Input: part model. Units: mm. Frame: model coordinates. Coordinates: 2 decimals unless noted, no trailing zeros. Loops run counter-clockwise (first coordinate to the right, second up) from the corner with the lowest first, then second, coordinate; pieces in that order, holes last.
```python
from build123d import *

# Parameters (mm, degrees)
BOSS_EXTRUDE1_DEPTH = 300
SKETCH3_R           = 2.25
CUT_EXTRUDE1_DEPTH  = 300
SKETCH6_R           = 2.25
CUT_EXTRUDE2_DEPTH  = 10
SKETCH8_R           = 2.25
CUT_EXTRUDE3_DEPTH  = 10


with BuildPart() as part:
    # Sketch1 → Boss-Extrude1 (new body)
    with BuildSketch(Plane(origin=(0, 0, 0), x_dir=(1, 0, 0), z_dir=(0, 1, 0))):
        Polygon((0, 0), (12.7, 0), (12.7, 2), (2, 2), (2, 12.7), (0, 12.7), align=None)
    extrude(amount=BOSS_EXTRUDE1_DEPTH)

    # Sketch3 → Cut-Extrude1 (cut)
    with BuildSketch(Plane(origin=(0, 0, -2), x_dir=(-1, 0, 0), z_dir=(0, 0, -1))):
        with Locations((-7.35, 275)):
            Circle(SKETCH3_R)
        with Locations((-7.35, 175)):
            Circle(SKETCH3_R)
        with Locations((-7.35, 75)):
            Circle(SKETCH3_R)
    extrude(amount=-CUT_EXTRUDE1_DEPTH, mode=Mode.SUBTRACT)

    # Sketch6 → Cut-Extrude2 (cut)
    with BuildSketch(Plane(origin=(2, 0, 0), x_dir=(0, 0, -1), z_dir=(1, 0, 0))):
        with Locations((7.35, 225)):
            Circle(SKETCH6_R)
        with Locations((7.35, 125)):
            Circle(SKETCH6_R)
        with Locations((7.35, 25)):
            Circle(SKETCH6_R)
    extrude(amount=-CUT_EXTRUDE2_DEPTH, mode=Mode.SUBTRACT)

    # Sketch8 → Cut-Extrude3 (cut)
    with BuildSketch(Plane.XY):
        with Locations((7.94, 253.6)):
            Circle(SKETCH8_R)
        with Locations((7.35, 25)):
            Circle(SKETCH8_R)
    extrude(amount=-CUT_EXTRUDE3_DEPTH, mode=Mode.SUBTRACT)


solid = part.part
```
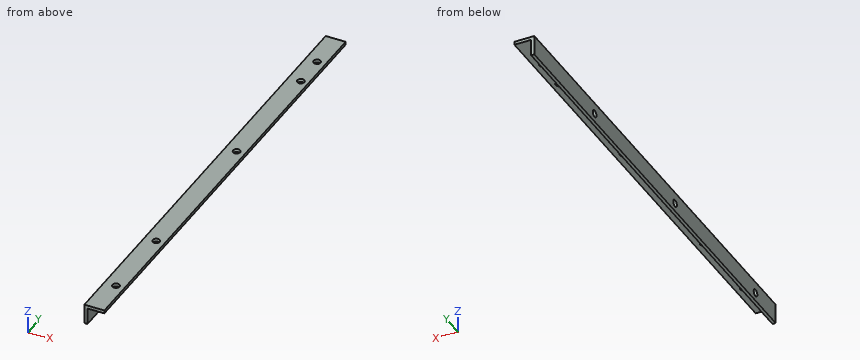
Item 1: Section query A-A (z = -7.35). Output: boundary loops of the cut face in (x, y).
Result:
outline: (0, 0) - (2, 0) - (2, 22.75) - (0, 22.75) - close; (0, 27.25) - (2, 27.25) - (2, 122.75) - (0, 122.75) - close; (0, 127.25) - (2, 127.25) - (2, 222.75) - (0, 222.75) - close; (0, 227.25) - (2, 227.25) - (2, 300) - (0, 300) - close
Item 2: Section query B-B (y = 51). Output: boundary loops of the cut face in (x, z).
Result:
outline: (0, -12.7) - (2, -12.7) - (2, -2) - (12.7, -2) - (12.7, 0) - (0, 0) - close
Item 3: Contact query for flat-ended pins moving along their axis: P1, Ø3, axis at x = 4, z = -10.5, coming from the -Y side; P2, Ø5, axis at x = 7.35, y = 25, coming from the -Z side; P3, Ø5, axis at y = 69, z = -7.5, coming from the +X side. Output: stop coordinate, or through.
Result:
P1: passes through
P2: stops at z = -2
P3: stops at x = 2
Item 4: Line query: L1, parallel to Y at x = 0.5, z = -7.35; L2, parallel to Y at x = 7.35, z = -0.6; L3, parallel to Y at x = 8.75, z = -0.5. Output: solid intervals per line, ascending.
Result:
L1: y = 0 to 22.75, 27.25 to 122.75, 127.25 to 222.75, 227.25 to 300
L2: y = 0 to 22.75, 27.25 to 72.75, 77.25 to 172.75, 177.25 to 251.43, 255.77 to 272.75, 277.25 to 300
L3: y = 0 to 23.24, 26.76 to 73.24, 76.76 to 173.24, 176.76 to 251.5, 255.7 to 273.24, 276.76 to 300
